Build history of the part. All positions in model axes, mm. A direction names the side the tool comes from. Give positions to 0.01 mm unless a question says otherwise; leave off trailing zeros. Loops run counter-clockwise (first coordinate to the right, second up) from the corner with the lowest first, then second, coordinate; pieces in that order, holes last. Notation, with made-up numbers: (-32.75, 87) -> (16.25, 87) arc R15 ccw to (16.25, 91) -> close; hole circle Ø1 at (63.25, 58). An arc over 180 degrees is marked (long way). Answer as a JSON object with one key per item and string values. Group by question number.
from build123d import *

# Parameters (mm, degrees)
SKETCH1_R           = 1.075
SKETCH1_W           = 50
SKETCH1_H           = 15
BOSS_EXTRUDE1_DEPTH = 8
SKETCH2_R           = 4.15
CUT_EXTRUDE1_DEPTH  = 2.5
FILLET1_R           = 7
FILLET2_R           = 7
FILLET3_R           = 7
FILLET4_R           = 7
FILLET5_R           = 7


with BuildPart() as part:
    # Sketch1 → Boss-Extrude1 (new body)
    # profile 1 of 4: a face of its own
    with BuildSketch(Plane(origin=(0, 0, 0), x_dir=(1, 0, 0), z_dir=(0, 1, 0))):
        with BuildLine():
            Line((-5, -8.077747211), (-5, -37))
            Line((-5, -37), (5, -37))
            Line((5, -37), (5, -8.077747211))
            ThreePointArc((5, -8.077747211), (0, -9.5), (-5, -8.077747211))
        make_face()
    # profile 2 of 4: a face of its own
    with BuildSketch(Plane(origin=(0, 0, 0), x_dir=(1, 0, 0), z_dir=(0, 1, 0))):
        with BuildLine():
            Line((-5, -3.665539315), (-5, -8.077747211))
            ThreePointArc((-5, -8.077747211), (0, -9.5), (5, -8.077747211))
            Line((5, -8.077747211), (5, -3.665539315))
            ThreePointArc((5, -3.665539315), (4.987177826, -3.5), (5, -3.334460685))
            Line((5, -3.334460685), (5, 0))
            Line((5, 0), (-5, 0))
            Line((-5, 0), (-5, -3.334460685))
            ThreePointArc((-5, -3.334460685), (-4.990388163, -3.416982422), (-4.987177826, -3.5))
            ThreePointArc((-4.987177826, -3.5), (-4.990388163, -3.583017578), (-5, -3.665539315))
        make_face()
        with Locations(Location((-3.5, -6.062177826, 0), (0, 0, 270))):
            Circle(SKETCH1_R, mode=Mode.SUBTRACT)
        with Locations(Location((0, -7, 0), (0, 0, 270))):
            Circle(SKETCH1_R, mode=Mode.SUBTRACT)
        with Locations(Location((3.5, -6.062177826, 0), (0, 0, 270))):
            Circle(SKETCH1_R, mode=Mode.SUBTRACT)
    # profile 3 of 4: a face of its own
    with BuildSketch(Plane(origin=(0, 0, 0), x_dir=(1, 0, 0), z_dir=(0, 1, 0))):
        with BuildLine():
            ThreePointArc((9.5, 0), (-4.623310502, 8.299096336), (-5, -8.077747211))
            Line((-5, -8.077747211), (-5, -3.665539315))
            ThreePointArc((-5, -3.665539315), (-7.137177826, -3.5), (-5, -3.334460685))
            Line((-5, -3.334460685), (-5, 0))
            Line((-5, 0), (5, 0))
            Line((5, 0), (5, -3.334460685))
            ThreePointArc((5, -3.334460685), (6.145195405, -2.428210337), (7.137177826, -3.5))
            ThreePointArc((7.137177826, -3.5), (6.145195405, -4.571789663), (5, -3.665539315))
            Line((5, -3.665539315), (5, -8.077747211))
            ThreePointArc((5, -8.077747211), (8.299096336, -4.623310502), (9.5, 0))
        make_face()
        with Locations(Location((-7, 0, 0), (0, 0, 270))):
            Circle(SKETCH1_R, mode=Mode.SUBTRACT)
        with Locations(Location((-6.062177826, 3.5, 0), (0, 0, 270))):
            Circle(SKETCH1_R, mode=Mode.SUBTRACT)
        with Locations(Location((-3.5, 6.062177826, 0), (0, 0, 270))):
            Circle(SKETCH1_R, mode=Mode.SUBTRACT)
        with Locations(Location((7, 0, 0), (0, 0, 270))):
            Circle(SKETCH1_R, mode=Mode.SUBTRACT)
        with Locations(Location((0, 7, 0), (0, 0, 270))):
            Circle(SKETCH1_R, mode=Mode.SUBTRACT)
        with Locations(Location((3.5, 6.062177826, 0), (0, 0, 270))):
            Circle(SKETCH1_R, mode=Mode.SUBTRACT)
        with Locations(Location((6.062177826, 3.5, 0), (0, 0, 270))):
            Circle(SKETCH1_R, mode=Mode.SUBTRACT)
    # profile 4 of 4: a face of its own
    with BuildSketch(Plane(origin=(0, 0, 0), x_dir=(1, 0, 0), z_dir=(0, 1, 0))):
        with Locations((-13, -44.5)):
            Rectangle(SKETCH1_W, SKETCH1_H)
    extrude(amount=BOSS_EXTRUDE1_DEPTH)

    # Sketch2 → Cut-Extrude1 (cut)
    with BuildSketch(Plane(origin=(0, 8, 0), x_dir=(1, 0, 0), z_dir=(0, 1, 0))):
        with Locations(Location((0, 0, 0), (0, 0, 270))):
            Circle(SKETCH2_R)
    extrude(amount=-CUT_EXTRUDE1_DEPTH, mode=Mode.SUBTRACT)

    # Fillet1
    fillet1_edges = [part.edges().sort_by_distance(p)[0] for p in [
        (5, 4, 37),
    ]]
    fillet(fillet1_edges, radius=FILLET1_R - 0.0001)  # a hair under: the kernel refuses the full size

    # Fillet2
    fillet2_edges = [part.edges().sort_by_distance(p)[0] for p in [
        (-5, 4, 37),
    ]]
    fillet(fillet2_edges, radius=FILLET2_R)

    # Fillet3
    fillet3_edges = [part.edges().sort_by_distance(p)[0] for p in [
        (-5, 4, 8.077747211),
        (5, 4, 8.077747211),
    ]]
    fillet(fillet3_edges, radius=FILLET3_R)

    # Fillet4
    fillet4_edges = [part.edges().sort_by_distance(p)[0] for p in [
        (12, 4, 37),
    ]]
    fillet(fillet4_edges, radius=FILLET4_R)

    # Fillet5
    fillet5_edges = [part.edges().sort_by_distance(p)[0] for p in [
        (-38, 4, 37),
    ]]
    fillet(fillet5_edges, radius=FILLET5_R)


solid = part.part
(1) Probe line 1 along X through (y, z) = (6.25, -3.5); line 2 along X through (y, z) = (6.5, 0) (3 decimals); line 3 along X through (y, z) = (6.5, 5.5). List the from-to ranges inside material, lowest first. Write a range as [from, to].
(2) Saw through at C-C on y = 1. Give the number of separate pieces and of enclosed holes in the cut face, plus the area to 3 significant figures.
(3) Saw through at B-B on x = -26.5. List the corners of the cut face in (y, z), plus the area to 3 significant figures.
(4) Saw through at A-A on z = 27. List the corners of the cut face in (x, y).
(5) 3-axis set-ups, long thin cutter, end or side, ignore diameter. For faces 1 (the flat face through (-22, 4, 37)), 2 (the cylindrical face through (-5.481, 4.056, 8.774)), 3 (the cylindrical face through (5.509, 4.056, 8.705)), 4 (the flat face through (0, 5.5, 0)): which of +Z, -Z, +X, -X, +Y, -Y reach the whole face in a straight line?
(6) Pull direction X, two halves, no side cores. Call faces 5 (the flat face through (-2, 8, 34)), 6 (the cylindrical face through (0.323, 3.944, -5.975)), 7 (the flat face through (-5, 4, 21)), 8 (the cylindrical face through (-3.18, 3.94, 7.09)): pulls with the +X half, pulls with the -X half, needs draft (parallel to the pull), parting line crosses it, or undercut.
(7) Pin check, flat tip, straight feed: pin 1 (1.7 mm diameter, centred on x = -3.5, z = -6.06, fed in from -Y). Stop position of the tip, or through.
Calculated:
{
 "1": {"line 1": "x = [-8.83, -7.14], [-4.99, -2.23], [2.23, 4.99], [7.14, 8.83]", "line 2": "x = [-9.5, -8.075], [-5.925, -4.15], [4.15, 5.925], [8.075, 9.5]", "line 3": "x = [-7.75, -4.42], [-2.58, 2.58], [4.42, 7.75]"},
 "2": {"separate pieces": "1", "enclosed holes": "12", "area": "1,280 mm^2"},
 "3": {"outline": "(0, 37) -> (8, 37) -> (8, 52) -> (0, 52) -> close", "area": "120 mm^2"},
 "4": {"outline": "(-5, 0) -> (5, 0) -> (5, 8) -> (-5, 8) -> close"},
 "5": {"face 1": "-Z, -X, +Y, -Y", "face 2": "-X, +Y, -Y", "face 3": "+X, +Y, -Y", "face 4": "+Y"},
 "6": {"face 5": "needs draft", "face 6": "undercut", "face 7": "pulls with the -X half", "face 8": "undercut"},
 "7": {"pin 1": "passes through"}
}
